Source: CAD feature listing. Evaluate the final solid. Frame: model axes, mm. A direction names the side the tool comes from. Round coordinates to 2 decimals unless told otherwise and drop trailing zeros. Order: outer loops, then holes, each group sorted by start corner. A loop starts at its lowest first (then second) coordinate and runs counter-clockwise, first axis right, second up. Notation, with made-up numbers: (23.25, -15.75) - (66.25, -15.75) arc R22 ccw to (66.25, 12.25) - close; hole circle Ø8 at (22, 6.5). An arc over 180 degrees is marked (long way). Return JSON: item names as keys, results as strings. Group by question number.
1) Ray query, line 1 (X direction, y = 1.85, z = -40.5); line 2 (Y direction, x = 8.75, z = -35); line 3 (Z direction, x = 5, y = 3.25). Return the intervals inside material, ascending. Write a range as from..to.
2) Section B-B, the plane y = 0.75. Return loops of the section in (x, z).
3) Access query for faces 1 (the cylindrical face through (5.9, 5.96, -2.58)), 2 (the flat face through (8, 1, -9)), 3 (the flat face through (8, 1, -72)), 4 (the flat face through (10.486, 1.521, -48.112)). Directions: +Z, -Z, +X, -X, +Y, -Y. A direction counts if a zero-diameter tool reaches every point of the face in a straight line with its end or side. Return the directions, or none.
4) Mould query, pull axis Z, two halves, no side actions, for faces 5 (the flat face through (15.3, 1.52, -29.24)), 6 (the flat face through (8, 2, -56)), 7 (the flat face through (9, 0, -37)), 8 (the flat face through (15.507, 1.521, -51.45)). Classes: pulls with the +Z half, pulls with the -Z half, needs draft (parallel to the pull), parting line crosses it, or undercut.
5) Section A-A, the plane z = -2.5. Return loops of the section in (x, y), plus the area to 3 significant figures.
6) Section D-D, the plane y = 5.75. Return loops of the section in (x, z), plus the area to 3 significant figures.
7) Section C-C, the plane x = 4. Return loops of the section in (y, z), plus the area to 3 significant figures.
8) Contact query for flat-ended pins moving along their axis: P1, Ø8, axis at x = 18, z = -21.5, coming from the +Y side; P2, Ø2, axis at x = 10.98, z = -40.5, coming from the +Y side; P3, Ø1.5, axis at y = 1.5, z = -11.5, coming from the +X side; P4, Ø0.8, axis at y = 2, z = -24.5, coming from the +X side. Output: stop coordinate, or through.
Autodesk Inventor part; units mm, degrees
ref_plane "YZ Plane" through (0, 0, 0) normal (1, 0, 0) x (0, 1, 0)
ref_plane "XZ Plane" through (0, 0, 0) normal (0, 1, 0) x (-1, 0, 0)
ref_plane "XY Plane" through (0, 0, 0) normal (0, 0, 1) x (1, 0, 0)
sketch "Sketch1" plane through (0, 0, 0) normal (0, 1, 0) x (-1, 0, 0)
  line L0 (0, 0) -> (0, -81)
  line L1 (0, -81) -> (-8, -81)
  line L2 (-8, -81) -> (-8, 0)
  line L3 (0, 0) -> (-8, 0)
  line L4 (-4, 0) -> (-4, -2.5)
  line L5 (-4, -81) -> (-4, -78.5)
  circle A0 centre (-4, -2.5) radius 1.9
  circle A1 centre (-4, -78.5) radius 1.9
  dimension "d0" = 81
  dimension "d1" = 8
  dimension "d2" = 81
  dimension "d3" = 2.5
  dimension "d4" = 2.5
  dimension "d5" = 3.8
  dimension "d6" = 3.8
extrude "Extrusion1" add sketch "Sketch1" along normal blind 3
extrude "Extrusion2" add sketch "Sketch1" along normal blind 9 contours A0 | A1
sketch "Sketch2" plane through (0, 3, 0) normal (0, 1, 0) x (1, 0, 0)
  line L0 (8, 0) -> (8, 81)
  line L1 (8, 40.5) -> (18, 40.5)
  line L2 (8, 40.5) -> (8, 25.5)
  line L3 (8, 25.5) -> (0, 25.5)
  line L4 (0, 81) -> (0, 0)
  line L5 (8, 40.5) -> (8, 55.5)
  line L6 (8, 55.5) -> (0, 55.5)
  line L7 (0, 55.5) -> (0, 25.5)
  line L8 (8, 25.5) -> (18, 40.5)
  line L9 (8, 55.5) -> (18, 40.5)
  line L10 (8.8321, 24.9453) -> (18.8321, 39.9453)
  line L11 (8.8321, 56.0547) -> (18.8321, 41.0547)
  line L12 (8.8321, 24.9453) -> (8, 23.6972)
  line L13 (8, 23.6972) -> (8, 25.5)
  line L14 (8, 55.5) -> (8, 57.3028)
  line L15 (8.8321, 56.0547) -> (8, 57.3028)
  line L16 (18.8321, 39.9453) -> (19.2019, 40.5)
  line L17 (18.8321, 41.0547) -> (19.2019, 40.5)
  line L18 (5, 25.5) -> (5, 13.7889)
  line L19 (5, 13.7889) -> (11.3282, 23.2812)
  line L20 (11.3282, 23.2812) -> (21.3282, 38.2812)
  line L21 (21.3282, 38.2812) -> (22.8074, 40.5)
  line L22 (22.8074, 40.5) -> (21.3282, 42.7188)
  line L23 (21.3282, 42.7188) -> (11.3282, 57.7188)
  line L24 (11.3282, 57.7188) -> (5, 67.2111)
  line L25 (5, 67.2111) -> (5, 55.5)
  line L26 (8, 23.6972) -> (0, 23.6972)
  line L27 (0, 25.5) -> (0, 23.6972)
  line L28 (8, 57.3028) -> (0, 57.3028)
  line L29 (0, 57.3028) -> (0, 55.5)
  point P0 (8, 18.2889)
  point P1 (8, 62.7111)
  dimension "d11" = 10
  dimension "d12" = 15
  dimension "d13" = 15
  dimension "d14" = 1
  dimension "d15" = 1
  dimension "d16" = 3
extrude "Extrusion3" add sketch "Sketch2" against normal blind 3 contours L12 L10 L16 L17 L11 L15 L0 L24 L23 L22 L21 L20 L19
extrude "Extrusion4" cut sketch "Sketch2" against normal blind 3 contours L26 L18 L3 L0 | L3 L4 L6 L0 | L26 L4 L3 L18 | L6 L25 L28 L0 | L6 L4 L28 L25
chamfer "Chamfer1" distance 3 angle 45 2 edges at (0, 1.5, -57.3028) (0, 1.5, -23.6972)
fillet "Fillet1" radius 1 2 edges at (8, 1.5, -57.3028) (8, 1.5, -23.6972)
sketch "Sketch3" plane through (0, 3, 0) normal (0, 1, 0) x (1, 0, 0)
  line L0 (22.8074, 40.5) -> (8, 62.7111)
  line L1 (22.8074, 40.5) -> (21.0044, 40.5)
  circle A0 centre (21.0044, 40.5) radius 0.4
  point P0 (0, 0)
  dimension "d25" = 1.803
  dimension "d26" = 0.8
extrude "Extrusion5" cut sketch "Sketch3" against normal blind 3
sketch "Sketch4" plane through (0, 3, 0) normal (0, 1, 0) x (1, 0, 0)
  line L0 (0, 57.3028) -> (8.0349, 57.3028)
  line L1 (0, 57.3028) -> (0, 23.6972)
  line L2 (0, 23.6972) -> (8.0349, 23.6972)
  line L3 (8.0349, 23.6972) -> (8.0349, 57.3028)
  line L4 (0, 60.3028) -> (3, 57.3028)
  line L5 (0, 57.3028) -> (0, 60.3028)
  line L6 (0, 60.3028) -> (3, 57.3028)
  line L7 (0, 20.6972) -> (0, 0)
  line L8 (0, 20.6972) -> (0, 23.6972)
  line L9 (0, 20.6972) -> (3, 23.6972)
  line L10 (0, 57.3028) -> (8, 57.3028)
  line L11 (8, 57.3028) -> (8, 55.5125)
  line L12 (8, 55.5125) -> (0, 55.5125)
  line L13 (0, 55.5125) -> (0, 57.3028)
  line L14 (8, 55.5125) -> (13.0424, 40.5013)
  line L15 (13.0424, 40.5013) -> (8.0349, 25.4511)
  line L16 (4.5889, 24.5965) -> (9.8792, 40.4967)
  line L17 (9.8792, 40.4967) -> (4.5467, 56.3715)
  circle A0 centre (10.9842, 40.4967) radius 0.75
  line L18 (9.8792, 40.4967) -> (8.0349, 40.5)
  line L19 (9.8792, 40.4967) -> (10.9842, 40.4967)
  point P0 (8.0349, 45.9872)
  point P1 (8.0349, 34.9536)
  dimension "d29" = 8
  dimension "d30" = 3
  dimension "d31" = 1.5
  dimension "d36" = 1.8443
  dimension "d37" = 1.105
extrude "Extrusion6" add sketch "Sketch4" against normal blind 3 contours L5 L4 L0 | L0 L11 L12 L1 | L12 L17 L3 L2 L1 | L2 L9 L8 | L12 L14 L3 L17 | L3 L14 L15 L16 L17
sketch "Sketch5" plane through (0, 3, 0) normal (0, 1, 0) x (1, 0, 0)
  line L0 (8.0349, 45.9872) -> (8.0349, 34.9536)
  line L1 (8.0349, 34.9536) -> (0.9671, 13.7113)
  line L2 (9.8792, 40.4967) -> (8.0349, 34.9536)
  line L3 (9.8792, 40.4967) -> (8.0349, 45.9872)
  line L4 (9.8792, 40.4967) -> (0.9671, 67.0279)
  line L5 (0.9671, 67.0279) -> (0.9671, 13.7113)
  line L6 (0, 81) -> (0, 0)
  line L7 (8.0349, 45.9872) -> (8.0349, 34.9536)
  point P0 (8.0349, 45.9872)
extrude "Extrusion7" cut sketch "Sketch5" against normal blind 3 contours L0 L1 L5 L4
sketch "Sketch6" plane through (0, 3, 0) normal (0, 1, 0) x (1, 0, 0)
  line L0 (9.8792, 40.4967) -> (0.9671, 67.0279)
  line L1 (0.9671, 67.0279) -> (0, 68.0001)
  line L2 (0, 81) -> (0, 0)
  line L3 (9.8792, 40.4967) -> (0.9671, 13.7113)
  line L4 (0.9671, 13.7113) -> (0, 10.8046)
  line L5 (0.9671, 13.7113) -> (0.9671, 67.0279)
  line L6 (0, 68.0001) -> (0, 10.8046)
  point P0 (0, 63.7751)
  point P1 (0, 17.0581)
extrude "Extrusion8" cut sketch "Sketch6" against normal blind 3 contours L5 L4 L2 L1
properties part number "SteeringBaru"
Geometry check:
{
 "1": {"line 1": "9.88..10.23, 11.73..13.04, 19.2..20.6, 21.4..22.81", "line 2": "0..3", "line 3": "-80.12..-76.88, -4.12..-0.88"},
 "2": {"outline": "(0, -81) - (8, -81) - (8, -62.71) - (22.81, -40.5) - (8, -18.29) - (8, 0) - (0, 0) - (0, -10.8) - (0.97, -13.71) - (8.03, -34.95) - (9.88, -40.5) - (8.03, -45.99) - (0.97, -67.03) - (0, -68) - close; hole (8, -57.15) arc R1 ccw to (8.3, -56.86) - (8.83, -56.05) - (19.2, -40.5) - (8.83, -24.95) - (8.3, -24.14) arc R1 ccw to (8.03, -23.88) - (8.03, -25.45) - (13.04, -40.5) - (8, -55.51) - close; hole circle Ø1.5 at (10.98, -40.5); hole circle Ø0.8 at (21, -40.5)"},
 "3": {"face 1": "+Y", "face 2": "+Z, +X, +Y, -Y", "face 3": "-Z, +X, +Y, -Y", "face 4": "+Y, -Y"},
 "4": {"face 5": "pulls with the +Z half", "face 6": "undercut", "face 7": "needs draft", "face 8": "pulls with the -Z half"},
 "5": {"outline": "(0, 0) - (8, 0) - (8, 3) - (5.9, 3) - (5.9, 9) - (2.1, 9) - (2.1, 3) - (0, 3) - close", "area": "46.8 mm2"},
 "6": {"outline": "circle Ø3.8 at (4, -78.5); circle Ø3.8 at (4, -2.5)", "area": "22.7 mm2"},
 "7": {"outline": "(0, -81) - (3, -81) - (3, -80.4) - (9, -80.4) - (9, -76.6) - (3, -76.6) - (3, -58) - (0, -58) - close; (0, -22.83) - (3, -22.83) - (3, -4.4) - (9, -4.4) - (9, -0.6) - (3, -0.6) - (3, 0) - (0, 0) - close", "area": "183 mm2"},
 "8": {"P1": "through", "P2": "y = 3", "P3": "x = 8", "P4": "x = 12.41"}
}
